Could you check a few things on this model? Use its own coordinates, in mm. A direction names the side the tool comes from. Give positions to 0.01 mm unless a question says otherwise; leave off trailing zeros. Loops run counter-clockwise (first coordinate to the right, second up) from the corner with the lowest first, then second, coordinate; pieces in that order, holes last. Notation, with made-up numbers: (56, -26.5) - (83, -26.5) arc R35 cw to (83, 6.5) - close; hole circle Ø2 at (46.25, 33.25). An arc over 180 degrees is marked (long way). One line per item, written item: value. Start each with the question number.
Q1. If we mould it in two halves opening along Z, with no side actions, what happens to faces 4 (the face through (-81.2, 3, -86)), 5 (the face through (-116.2, 2, -160)), 6 (the face through (-59, 2, -199)), 7 (the face through (-78, 2, -5))? For each: released by +Z, released by -Z, zero draft, split by the parting line, or undercut.
Q2. I want a section at A-A (z = 1). Please give me the cut outline in (x, y).
Q3. I want a section at B-B (y = 2.25). Count the separate pieces of the cut face and the enclosed holes in it, then the cut area to 3 significant figures.
Q4. If I drill on line 1 (Z direction, x = -25.5, y = 4.55); line 2 (Z direction, x = -32, y = 3.85); line 3 (Z direction, x = -56.2, y = 1.9), over which ranges is the centre line in solid material (lowest first)? Write a range as from..to.
Q5. For faces 1 (the face through (-40, 2, 14)), 2 (the face through (-80.059, 2.465, -134.497)), 3 (the face through (-121.2, 2, -96)), which set-ups out of +Z, -Z, +X, -X, +Y, -Y let a thin tool reach every point of the face, with its end or its side?
Q6. I'm going to push flat-ended pins straight in: P1, Ø1.5, axis at x = -80, y = 2.5, coming from the +Z side; P2, Ø10, axis at x = -52.5, z = 0.5, coming from the -Y side; P3, Ø1.5, axis at y = 3, z = -31.5, coming from the -X side; P4, Ø1.5, axis at y = 1.5, z = -74, coming from the +X side. Where does each tip first touch, or does it pass through?
Q7. I want a section at C-C (x = -98.5). Please give me the cut outline in (y, z).
Autodesk Inventor part; units mm, degrees
ref_plane "YZ Plane" through (0, 0, 0) normal (1, 0, 0) x (0, 1, 0)
ref_plane "XZ Plane" through (0, 0, 0) normal (0, 1, 0) x (-1, 0, 0)
ref_plane "XY Plane" through (0, 0, 0) normal (0, 0, 1) x (1, 0, 0)
sketch "Sketch1" plane through (0, 0, 0) normal (0, 1, 0) x (-1, 0, 0)
  line L0 (40, -5) -> (116.2, -5)
  line L1 (116.2, -199) -> (0, -199)
  line L2 (0, -199) -> (0, 0)
  line L3 (40, -5) -> (40, 35)
  line L4 (40, 35) -> (0, 35)
  line L5 (0, 35) -> (0, 0)
  line L6 (116.2, -71.25) -> (121.2, -71.25)
  line L7 (121.2, -71.25) -> (121.2, -121.25)
  line L8 (121.2, -121.25) -> (116.2, -121.25)
  line L9 (116.2, -5) -> (116.2, -71.25)
  line L10 (116.2, -121.25) -> (116.2, -199)
  dimension "d0" = 116.2
  dimension "d6" = 77.75
  dimension "d8" = 50
  dimension "d9" = 5
  dimension "d11" = 40
  dimension "d12" = 40
  dimension "d31" = 194
extrude "Extrusion1" add sketch "Sketch1" along normal blind 5
sketch "Sketch2" plane through (0, 5, 0) normal (0, 1, 0) x (1, 0, 0)
  line L0 (-32, -64.6005) -> (-32, 40.6005) construction
  line L1 (-139.7989, 191) -> (-75.0444, 191) construction
  line L2 (0, 199) -> (-116.2, 199)
  line L3 (-116.2, 199) -> (-116.2, 121.25)
  line L4 (-116.2, 5) -> (-40, 5)
  line L5 (-40, 5) -> (-40, -35)
  point P0 (0, 0)
  point P1 (-32, -24)
  point P2 (-32, -12)
  point P3 (-104.2, 191)
  point P4 (-73.2, 191)
  point P5 (-32, -12)
  dimension "d16" = 31
  dimension "d17" = 8
  dimension "d18" = 12
  dimension "d19" = 17
  dimension "d20" = 12
  dimension "d21" = 8
hole "Hole1" at (-32, 5, 24) at (-32, 5, 12) at (-104.2, 5, -191) at (-73.2, 5, -191) direction (0, -1, 0) diameter 3.8 end through all
fillet "Fillet1" radius 2 2 edges at (-40, 2.5, 35) (0, 2.5, 35)
sketch "Sketch3" plane through (0, 5, 0) normal (0, 1, 0) x (1, 0, 0)
  line L0 (-56.2, 96.1981) -> (-56.2, 272.5509) construction
  line L1 (-116.2, 199) -> (-116.2, 121.25)
  line L2 (0, 199) -> (-116.2, 199)
  point P0 (0, 0)
  point P1 (-56.2, 187)
  point P2 (-56.2, 175)
  dimension "d32" = 60
  dimension "d33" = 12
  dimension "d34" = 12
hole "Hole2" at (-56.2, 5, -187) at (-56.2, 5, -175) direction (0, -1, 0) diameter 3.8 end through all
sketch "Sketch5" plane through (0, 5, 0) normal (0, 1, 0) x (1, 0, 0)
  line L0 (0, -33) -> (0, 199)
  line L1 (0, 170.75) -> (-42, 170.75)
  line L2 (-44, 168.75) -> (-44, 167.7)
  line L3 (-42, 165.7) -> (0, 165.7)
  line L4 (0, 165.7) -> (0, 170.75)
  line L5 (0, 199) -> (-116.2, 199)
  arc A0 (-44, 167.7) -> (-42, 165.7) centre (-42, 167.7) ccw
  arc A1 (-42, 170.75) -> (-44, 168.75) centre (-42, 168.75) ccw
  point P0 (0, 0)
  point P1 (-44, 165.7)
  point P2 (-44, 170.75)
  point P3 (0, 165.7)
  dimension "d47" = 44
  dimension "d48" = 5.05
  dimension "d49" = 33.3
  dimension "d50" = 2
extrude "Extrusion3" cut sketch "Sketch5" against normal blind 5
sketch "Sketch6" plane through (0, 5, 0) normal (0, 1, 0) x (1, 0, 0)
  line L0 (-135.5788, 175.75) -> (79.5788, 175.75) construction
  line L1 (0, 199) -> (-116.2, 199) construction
  line L2 (0, 170.75) -> (0, 199) construction
  point P0 (0, 0)
  point P1 (-16, 175.75)
  point P2 (-28, 175.75)
  point P3 (-73.5, 175.75)
  dimension "d53" = 23.25
  dimension "d54" = 16
  dimension "d55" = 28
  dimension "d56" = 73.5
hole "Hole3" at (-16, 5, -175.75) at (-28, 5, -175.75) at (-73.5, 5, -175.75) direction (0, -1, 0) diameter 3.8 end through all
sketch "Sketch7" plane through (0, 5, 0) normal (0, 1, 0) x (1, 0, 0)
  line L0 (-6.5, 43.9272) -> (-6.5, -51.0616) construction
  line L1 (0, -33) -> (0, 165.7)
  line L2 (-38, -35) -> (-2, -35)
  point P0 (0, 0)
  point P1 (-6.5, -21)
  dimension "d64" = 6.5
  dimension "d65" = 14
hole "Hole4" at (-6.5, 5, 21) direction (0, -1, 0) diameter 3.8 end through all
sketch "Sketch8" plane through (0, 5, 0) normal (0, 1, 0) x (1, 0, 0)
  line L0 (-129.4929, 178) -> (-73.5, 178) construction
  line L1 (0, 199) -> (-116.2, 199)
  line L2 (-88.7, 175) -> (-87.7, 175)
  line L3 (-85.2, 177.5) -> (-85.2, 178.5)
  line L4 (-87.7, 181) -> (-88.7, 181)
  line L5 (-91.2, 178.5) -> (-91.2, 177.5)
  line L6 (-91.2, 175) -> (-85.2, 181) construction
  line L7 (-85.2, 175) -> (-91.2, 181) construction
  line L8 (-116.2, 199) -> (-116.2, 121.25)
  arc A0 (-88.7, 181) -> (-91.2, 178.5) centre (-88.7, 178.5) ccw
  arc A1 (-91.2, 177.5) -> (-88.7, 175) centre (-88.7, 177.5) ccw
  arc A2 (-87.7, 175) -> (-85.2, 177.5) centre (-87.7, 177.5) ccw
  arc A3 (-85.2, 178.5) -> (-87.7, 181) centre (-87.7, 178.5) ccw
  point P0 (0, 0)
  point P1 (-88.2, 178)
  dimension "d73" = 21
  dimension "d74" = 6
  dimension "d75" = 6
  dimension "d76" = 25
  dimension "d77" = 2.5
extrude "Extrusion4" cut sketch "Sketch8" against normal through all
sketch "Sketch9" plane through (0, 5, 0) normal (0, 1, 0) x (1, 0, 0)
  line L0 (0, -33) -> (0, 165.7)
  line L1 (0, 135.7) -> (-81.2, 135.7)
  line L2 (-81.2, 135.7) -> (-81.2, 35)
  line L3 (-81.2, 35) -> (0, 35)
  line L4 (0, 35) -> (0, 135.7)
  line L5 (0, 165.7) -> (-42, 165.7)
  line L6 (-116.2, 5) -> (-40, 5)
  line L7 (-116.2, 199) -> (-116.2, 121.25)
  point P0 (0, 0)
  point P1 (0, 35)
  dimension "d80" = 30
  dimension "d81" = 30
  dimension "d82" = 35
extrude "Extrusion5" cut sketch "Sketch9" against normal through all
fillet "Fillet3" radius 4 4 edges at (-81.2, 2.5, -135.7) (-81.2, 2.5, -35) (0, 2.5, -35) (0, 2.5, -135.7)
properties part number "BAttery divider"
Worked answers:
1. face 4: undercut
1. face 5: zero draft
1. face 6: released by -Z
1. face 7: released by +Z
2. outline: (-40, 0) - (0, 0) - (0, 5) - (-40, 5) - close
3. separate pieces: 1
3. enclosed holes: 11
3. area: 15,800 mm²
4. line 1: z = -199..-170.75, -165.7..-135.7, -35..35
4. line 2: z = -199..-170.75, -165.7..-135.7, -35..10.1, 13.9..22.1, 25.9..35
4. line 3: z = -199..-188.9, -185.1..-176.9, -173.1..-135.7, -35..-5
5. face 1: +Z, -X, +Y, -Y
5. face 2: +X, +Y, -Y
5. face 3: +Z, -Z, -X, +Y, -Y
6. P1: stops at z = -5
6. P2: passes through
6. P3: stops at x = -116.2
6. P4: stops at x = -81.2
7. outline: (0, -199) - (5, -199) - (5, -5) - (0, -5) - close
